from build123d import *

# Parameters (mm, degrees)
SKETCH_1_W      = 22.6
SKETCH_1_H      = 12.4
EXTRUDE_1_DEPTH = 18
SKETCH_2_W      = 32.4
SKETCH_2_H      = 12.4
SKETCH_2_R      = 1.25
EXTRUDE_2_DEPTH = 3.4
SKETCH_3_W      = 22.6
SKETCH_3_H      = 12.4
EXTRUDE_3_DEPTH = 1.9
EXTRUDE_4_DEPTH = 6
SKETCH_5_R      = 2.25
EXTRUDE_5_DEPTH = 4.5


with BuildPart() as part:
    # 草图1 → 凸台-拉伸1 (new body)
    with BuildSketch(Plane(origin=(0, 0, 0), x_dir=(1, 0, 0), z_dir=(0, 1, 0))):
        Rectangle(SKETCH_1_W, SKETCH_1_H)
    extrude(amount=EXTRUDE_1_DEPTH)

    # 草图2 → 凸台-拉伸2 (add)
    with BuildSketch(Plane(origin=(0, 18, 0), x_dir=(1, 0, 0), z_dir=(0, 1, 0))):
        Rectangle(SKETCH_2_W, SKETCH_2_H)
        with Locations((-13.7, 0)):
            Circle(SKETCH_2_R, mode=Mode.SUBTRACT)
        with Locations((13.7, 0)):
            Circle(SKETCH_2_R, mode=Mode.SUBTRACT)
    extrude(amount=EXTRUDE_2_DEPTH)

    # 草图3 → 凸台-拉伸3 (add)
    with BuildSketch(Plane(origin=(0, 21.4, 0), x_dir=(1, 0, 0), z_dir=(0, 1, 0))):
        Rectangle(SKETCH_3_W, SKETCH_3_H)
    extrude(amount=EXTRUDE_3_DEPTH)

    # 草图4 → 凸台-拉伸4 (add)
    with BuildSketch(Plane(origin=(0, 23.3, 0), x_dir=(1, 0, 0), z_dir=(0, 1, 0))):
        with BuildLine():
            Line((1.659485126, 2.5), (-0.47750061, 2.5))
            ThreePointArc((-0.47750061, 2.5), (-11.3, 0), (-0.47750061, -2.5))
            Line((-0.47750061, -2.5), (1.659485126, -2.5))
            ThreePointArc((1.659485126, -2.5), (4.159485126, 0), (1.659485126, 2.5))
        make_face()
    extrude(amount=EXTRUDE_4_DEPTH)

    # 草图5 → 凸台-拉伸5 (add)
    with BuildSketch(Plane(origin=(0, 29.3, 0), x_dir=(1, 0, 0), z_dir=(0, 1, 0))):
        with Locations((-5.6, 0)):
            Circle(SKETCH_5_R)
    extrude(amount=EXTRUDE_5_DEPTH)


solid = part.part
Can you work these out from the model? Positions are in its coordinate system, mm. A direction names the side the tool comes from. Coordinates: 2 decimals unless noted, no trailing zeros. Loops run counter-clockwise (first coordinate to the right, second up) from the corner with the lowest first, then second, coordinate; pieces in that order, holes last. Notation, with made-up numbers: (49, -33) - (90, -33) arc R21 cw to (90, 6) - close; hole circle Ø3 at (-30, 74). An arc over 180 degrees is marked (long way). Put each result on its own line as item: value. Start each with the question number.
Item 1: If we mould it in two halves opening along Z, with no side actions, what happens to faces 1 (the face through (-12.545, 19.676, 0.479)), 2 (the face through (-13.8, 18, -1.5)), 3 (the face through (-11.296, 26.258, -0.214))? For each: +Z half, -Z half, draft (parallel to the pull), parting line (faces both ways), or undercut.
Item 2: Suppose I cut it at A-A (x = -13.7). Please give me the cut outline in (y, z), and give its area (3 significant figures).
Item 3: Suppose I cut it at D-D (y = 12.5). Please give me the cut outline in (x, z).
Item 4: Suppose I cut it at C-C (x = 0.5). Please give me the cut outline in (y, z), and give its area (3 significant figures).
Item 5: Which directions (+Z, -Z, +X, -X, +Y, -Y) give clear straight access to the entire face, cutting with the end or side of a thin tool? Please do faces 4 (the face through (1, 26, 2.5)), 5 (the face through (-13.8, 21.4, -1.5)), 6 (the face through (-2, 29.3, 0)), 7 (the face through (1, 26, -2.5)).
Item 6: If I drill on line 1 along X through (y, z) = (19, 0); line 2 along Z through (x, y) = (-13.7, 20.55); line 3 along Y through (x, z) = (9.5, -1), over which ranges is the centre line in solid material (lowest first)?
Item 7: Suppose I cut it at B-B (z = -0.5). State how many separate pieces and enclosed holes the cut face has, and give its area (3 significant figures).
Item 8: For pin 1 (1.5 mm diameter, centred on y = 5.5, z = 2.5, fed in from -X); pin 2 (1.7 mm diameter, centred on x = 0.5, y = 26.5, fed in from -Z); pin 3 (5.5 mm diameter, centred on x = -14, z = 1.5, fed in from +Y); pin 4 (2 mm diameter, centred on y = 22, z = 3, fed in from +X), each with a flat end and sliding along its axis, tell me the tip position at first contact or that it passes through.
Here are the results:
1. face 1: undercut
1. face 2: draft
1. face 3: parting line
2. outline: (18, -6.2) - (21.4, -6.2) - (21.4, -1.25) - (18, -1.25) - close; (18, 1.25) - (21.4, 1.25) - (21.4, 6.2) - (18, 6.2) - close
2. area: 33.7 mm²
3. outline: (-11.3, -6.2) - (11.3, -6.2) - (11.3, 6.2) - (-11.3, 6.2) - close
4. outline: (0, -6.2) - (23.3, -6.2) - (23.3, -2.5) - (29.3, -2.5) - (29.3, 2.5) - (23.3, 2.5) - (23.3, 6.2) - (0, 6.2) - close
4. area: 319 mm²
5. face 4: +Z, +X, +Y
5. face 5: +Z, -Z, -X, +Y
5. face 6: +Y
5. face 7: -Z, +X, +Y
6. line 1: -16.2 to -14.95, -12.45 to 12.45, 14.95 to 16.2
6. line 2: -6.2 to -1.25, 1.25 to 6.2
6. line 3: 0 to 23.3
7. separate pieces: 3
7. enclosed holes: 0
7. area: 656 mm²
8. pin 1: x = -11.3
8. pin 2: z = -2.5
8. pin 3: y = 23.3
8. pin 4: x = 16.2
